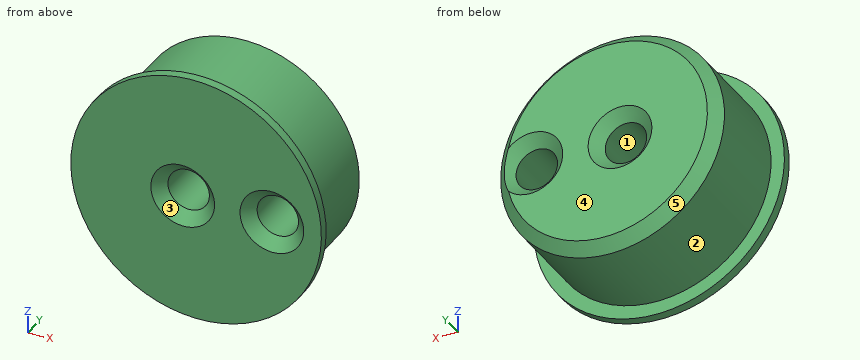
```python
from build123d import *
from build123d.topology import SkipClean

# Parameters (mm, degrees)
SKETCH_1_R      = 5.02
SKETCH_1_R_2    = 0.93
EXTRUDE_1_DEPTH = 4.4
EXTRUDE_START   = 0.4
SKETCH_3_R      = 5.62
SKETCH_3_R_2    = 0.93
EXTRUDE_2_DEPTH = 0.4
CHAMFER_1_SIZE  = 0.5


with BuildPart() as part:
    # 草图1 → 凸台-拉伸1 (new body)
    with BuildSketch(Plane(origin=(0, 0, 0), x_dir=(1, 0, 0), z_dir=(0, 1, 0))):
        with Locations(Location((0, 0, 0), (0, 0, 270))):
            Circle(SKETCH_1_R)
        with Locations(Location((3.4, 0, 0), (0, 0, 270))):
            Circle(SKETCH_1_R_2, mode=Mode.SUBTRACT)
        with Locations(Location((-0.6, 0, 0), (0, 0, 90))):
            Circle(SKETCH_1_R_2, mode=Mode.SUBTRACT)
    extrude(amount=EXTRUDE_1_DEPTH)

    # 草图3 → 凸台-拉伸2 (add)
    with SkipClean():  # the faces are left unmerged after this step: merging them gives an invalid solid
        with BuildSketch(Plane.XZ.offset(EXTRUDE_START)):
            with Locations(Location((0, 0, 0), (0, 0, 270))):
                Circle(SKETCH_3_R)
            with Locations(Location((3.4, 0, 0), (0, 0, 270))):
                Circle(SKETCH_3_R_2, mode=Mode.SUBTRACT)
            with Locations(Location((-0.6, 0, 0), (0, 0, 270))):
                Circle(SKETCH_3_R_2, mode=Mode.SUBTRACT)
        extrude(amount=-EXTRUDE_2_DEPTH)

    # 倒角1
    # the kernel refuses this chamfer: 0.5 mm, written as the material it takes off along each edge
    with BuildSketch(Plane(origin=(3.4, -0.4, 0), x_dir=(0, 0, -1), z_dir=(-1, 0, 0))) as chamfer_1_piece_1:
        Polygon((0.93 + CHAMFER_1_SIZE, 0), (0.93, -CHAMFER_1_SIZE), (0.93, 0), align=None)
    revolve(axis=Axis((3.4, -0.4, 0), (0, -1, 0)), mode=Mode.SUBTRACT)
    with BuildSketch(Plane(origin=(-0.6, -0.4, 0), x_dir=(0, 0, -1), z_dir=(-1, 0, 0))) as chamfer_1_piece_2:
        Polygon((0.93 + CHAMFER_1_SIZE, 0), (0.93, -CHAMFER_1_SIZE), (0.93, 0), align=None)
    revolve(axis=Axis((-0.6, -0.4, 0), (0, -1, 0)), mode=Mode.SUBTRACT)
    with BuildSketch(Plane(origin=(0, 4.4, 0), x_dir=(0, 0, 1), z_dir=(-1, 0, 0))) as chamfer_1_piece_3:
        Polygon((5.02, -CHAMFER_1_SIZE), (5.02 - CHAMFER_1_SIZE, 0), (5.02, 0), align=None)
    revolve(axis=Axis((0, 4.4, 0), (0, 1, 0)), mode=Mode.SUBTRACT)
    with BuildSketch(Plane(origin=(3.4, 4.4, 0), x_dir=(0, 0, 1), z_dir=(-1, 0, 0))) as chamfer_1_piece_4:
        Polygon((0.93 + CHAMFER_1_SIZE, 0), (0.93, -CHAMFER_1_SIZE), (0.93, 0), align=None)
    revolve(axis=Axis((3.4, 4.4, 0), (0, 1, 0)), mode=Mode.SUBTRACT)
    with BuildSketch(Plane(origin=(-0.6, 4.4, 0), x_dir=(0, 0, -1), z_dir=(1, 0, 0))) as chamfer_1_piece_5:
        Polygon((0.93 + CHAMFER_1_SIZE, 0), (0.93, -CHAMFER_1_SIZE), (0.93, 0), align=None)
    revolve(axis=Axis((-0.6, 4.4, 0), (0, 1, 0)), mode=Mode.SUBTRACT)


solid = part.part
```
Work out the finished part from the listing and answer in its coordinate system (mm). Face numbers are marked on the shaded views. A direction names the side the tool comes from. Coordinates: 2 decimals unless noted, no trailing zeros. Order: outer loops, then holes, each group sorted by start corner. A loop starts at its lowest first (then second) coordinate and runs counter-clockwise, first axis right, second up. Notation, with made-up numbers: M 71.25,46 L 89.25,46 A26 ccw 89.25,78 Z; hole C 53.5,-22 d4. An arc over 180 degrees is marked long. Use CSV: the item, a comma, the result in double quotes.
1) Consider line 1 (X direction, y = 2.95, z = 0); line 2 (Z direction, x = 3.4, y = 1.35); line 3 (Y direction, x = -4.25, z = 3.5). Determine where each line is inside the solid, lowest interval first. Write a range as [from, to].
Worked out:
line 1,"x = [-5.02, -1.53], [0.33, 2.47], [4.33, 5.02]"
line 2,"z = [-3.69, -0.93], [0.93, 3.69]"
line 3,"y = [-0.4, 0]"
2) Section A-A on y = 3.5 is taken. Write down the section's boundary in (x, z), plus the area to 3 significant figures.
Worked out:
outline,"C 0,0 d10.04; hole C -0.6,0 d1.86; hole C 3.4,0 d1.86"
area,"73.7 mm^2"
3) Section B-B on x = 5.25 is taken. Write down the section's boundary in (y, z).
Worked out:
outline,"M -0.4,-2.01 L 0,-2.01 L 0,2.01 L -0.4,2.01 Z"
4) Determine the mould class of the marked faces 3, 4 and 5 for opening direction Z: released by +Z, released by -Z, zero draft, split by the parting line, or undercut.
Worked out:
face 3,"undercut"
face 4,"zero draft"
face 5,"split by the parting line"
5) Flat-ended cylindrical pins translate along their axes: pin 1 Ø2 at (y, z) = (3.5, -3) entering from -X; pin 2 Ø2 at (x, z) = (3.4, 0) entering from +Y. Find the tip coordinate at first contact, or state that the pin passes through.
Worked out:
pin 1,"stops at x = -4.6"
pin 2,"stops at y = 3.97"
6) For the marked faces 1 and 2, determine the directions among +Z, -Z, +X, -X, +Y, -Y from which every point of the face is accessible in a straight line to the end or side of a thin tool.
Worked out:
face 1,"+Y, -Y"
face 2,"+Y"
